Design review of the part built by this model. Coordinates are the model's own, in mm. Face numbers are marked on the shaded views. Round coordinates to 2 decimals unless told otherwise and drop trailing zeros. Order: outer loops, then holes, each group sorted by start corner. A loop starts at its lowest first (then second) coordinate and runs counter-clockwise, first axis right, second up. Notation, with made-up numbers: M -37,2.25 L 20,2.25 A8 ccw 20,11.25 Z; hole C 44,23 d9. An arc over 180 degrees is marked long. Use a Markdown table: item, result. Add a question column.
(1) The part is to be moulded in two halves that separate along X. For the marked faces 1 and 2, say which applies: released by +X, released by -X, zero draft, split by the parting line, or undercut.
(2) Take a section at A-A (y = 18). Write out the cut boundary in (x, z).
(3) To check wall thickness, follow probe 1 along X at (y, z) = (1.3, -37.5); probe 2 along X at (y, z) = (31.1, -37.5); probe 3 along Z at (x, y) = (-17, 29.5). State the ranges of each line that lie inside material, in increasing order. Write a range as from..to.
(4) For pin 1 (2.5 mm diameter, centred on x = 0, z = -37.5, fed in from +Y); pin 2 (4 mm diameter, centred on x = -12, z = -9, fed in from +Y); pin 3 (8 mm diameter, centred on y = 16.5, z = -40, fed in from +X); pin 4 (8.5 mm diameter, centred on x = -0.5, z = -41.5, fed in from -Y), all flat-tipped, find the tip position at first contact; note any pin that passes through.
(5) Take a section at B-B (y = 28.5). Write out the cut boundary in (x, z).
```python
from build123d import *

# Parameters (mm, degrees)
FILLET_1_R = 13
FILLET_2_R = 13
FILLET_3_R = 3
FILLET_4_R = 3


with BuildPart() as part:
    # 草图1 → 旋转1 (revolve)
    with BuildSketch(Plane(origin=(0, 0, 0), x_dir=(0, 0, -1), z_dir=(1, 0, 0)), mode=Mode.PRIVATE) as revolve_1_sk:
        Polygon((25.5, 32), (35.5, 32), (35.5, 30), (37.5, 30), (37.5, 2), (35.5, 2), (35.5, 0), (25.5, 0), (25.5, 2), (23.5, 2), (23.5, 0), (13, 0), (13, 1), (12, 1), (12, 0), (0, 0), (0, 32), (12, 32), (12, 31), (13, 31), (13, 32), (23.5, 32), (23.5, 30), (25.5, 30), align=None)
    revolve(revolve_1_sk.sketch.rotate(Axis((0, 2, -37.5), (0, 1, 0)), 180), axis=Axis((0, 2, -37.5), (0, 1, 0)))

    # 圆角1
    # the kernel refuses this fillet: 13 mm, written as the material it takes off along each edge
    with BuildSketch(Plane(origin=(0, 0, -37.5), x_dir=(0, 0, -1), z_dir=(1, 0, 0))) as fillet_1_piece_1:
        with BuildLine():
            CenterArc((24.5, 12.961481397), FILLET_1_R, 274.411725786, 85.588274214)
            Line((37.5, 12.961481397), (37.76, 12.961481397))
            Line((37.76, 12.961481397), (37.76, 0))
            Line((37.76, 0), (37.5, -0.26))
            ThreePointArc((37.5, -0.26), (31.5, -0.26), (25.52, -0.259229628))
            Line((25.52, -0.259229628), (25.5, 0))
        make_face()
    revolve(axis=Axis((0, 0, -37.5), (0, 1, 0)), mode=Mode.SUBTRACT)
    with BuildSketch(Plane(origin=(0, 32, -37.5), x_dir=(0, 0, -1), z_dir=(1, 0, 0))) as fillet_1_piece_2:
        with BuildLine():
            CenterArc((24.5, -12.961481397), FILLET_1_R, 0, 85.588274214)
            Line((25.5, 0), (25.52, 0.259229628))
            ThreePointArc((25.52, 0.259229628), (31.5, 0.26), (37.5, 0.26))
            Line((37.5, 0.26), (37.76, 0))
            Line((37.76, 0), (37.76, -12.961481397))
            Line((37.76, -12.961481397), (37.5, -12.961481397))
        make_face()
    revolve(axis=Axis((0, 32, -37.5), (0, 1, 0)), mode=Mode.SUBTRACT)

    # 圆角2
    # the kernel refuses this fillet: 13 mm, written as the material it takes off along each edge
    with BuildSketch(Plane(origin=(0, 32, -37.5), x_dir=(0, 0, -1), z_dir=(1, 0, 0))) as fillet_2_piece_1:
        with BuildLine():
            CenterArc((19.5, -13), FILLET_2_R, 67.380135052, 22.619864948)
            Line((24.5, -1), (24.5, 0))
            Line((24.5, 0), (19.5, 0))
        make_face()
    revolve(axis=Axis((0, 32, -37.5), (0, 1, 0)), mode=Mode.SUBTRACT)
    with BuildSketch(Plane(origin=(0, 0, -37.5), x_dir=(0, 0, -1), z_dir=(1, 0, 0))) as fillet_2_piece_2:
        with BuildLine():
            CenterArc((19.5, 13), FILLET_2_R, 270, 22.619864948)
            Line((19.5, 0), (24.5, 0))
            Line((24.5, 0), (24.5, 1))
        make_face()
    revolve(axis=Axis((0, 0, -37.5), (0, 1, 0)), mode=Mode.SUBTRACT)

    # 圆角3
    # the kernel refuses this fillet: 3 mm, written as the material it takes off along each edge
    with BuildSketch(Plane(origin=(0, 32, -37.5), x_dir=(0, 0, -1), z_dir=(1, 0, 0))) as fillet_3_piece_1:
        with BuildLine():
            CenterArc((16.828427125, -3), FILLET_3_R, 90, 70.528779366)
            Line((16.828427125, 0), (16.828427125, 0.06))
            Line((16.828427125, 0.06), (14, 0.06))
            Line((14, 0.06), (13.94, 0))
            ThreePointArc((13.94, 0), (13.94, -1), (13.943431458, -1.98))
            Line((13.943431458, -1.98), (14, -2))
        make_face()
    revolve(axis=Axis((0, 32, -37.5), (0, 1, 0)), mode=Mode.SUBTRACT)

    # 圆角4
    # the kernel refuses this fillet: 3 mm, written as the material it takes off along each edge
    with BuildSketch(Plane(origin=(0, 32, -37.5), x_dir=(0, 0, -1), z_dir=(1, 0, 0))) as fillet_4_piece_1:
        with BuildLine():
            CenterArc((27.336484743, -3.372198092), FILLET_4_R, 73.521921674, 54.224042323)
            Line((28.187430166, -0.495413101), (28.204449075, -0.437877401))
            ThreePointArc((28.204449075, -0.437877401), (26.867646141, -0.117889541), (25.504615385, 0.059822222))
            Line((25.504615385, 0.059822222), (25.44, 0))
            ThreePointArc((25.44, 0), (25.44, -0.5), (25.463270305, -0.952556038))
            Line((25.463270305, -0.952556038), (25.5, -1))
        make_face()
    revolve(axis=Axis((0, 32, -37.5), (0, 1, 0)), mode=Mode.SUBTRACT)


solid = part.part
```
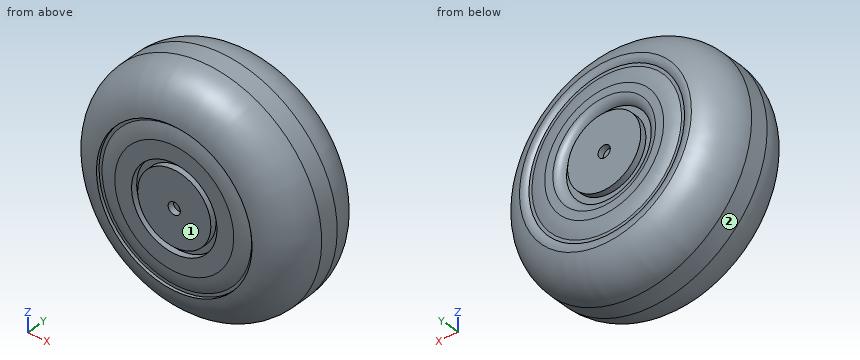
Verdict:
| question | item | result |
|---|---|---|
| 1 | face 1 | zero draft |
| 1 | face 2 | split by the parting line |
| 2 | outline | C 0,-37.5 d75 |
| 3 | probe 1 | x = -30.25..-14, -12..-2, 2..12, 14..30.25 |
| 3 | probe 2 | x = -29.35..-25.64, -24.25..-14.69, -12..-2, 2..12, 14.69..24.25, 25.64..29.35 |
| 3 | probe 3 | z = -64.87..-10.13 |
| 4 | pin 1 | stops at y = 30 |
| 4 | pin 2 | stops at y = 31.26 |
| 4 | pin 3 | stops at x = 37.5 |
| 4 | pin 4 | stops at y = 0 |
| 5 | outline | C 0,-37.5 d66.83 |
